Could you check a few things on this model? Use its own coordinates, in mm. A direction names the side the tool comes from. Give positions to 0.01 mm unless a question says otherwise; leave off trailing zeros. Loops run counter-clockwise (first coordinate to the right, second up) from the corner with the lowest first, then second, coordinate; pieces in that order, holes last.
1. For faces 1 (the cylindrical face through (-8.5, 4.2, -13)), 2 (the cylindrical face through (-0.1, 0.5, -11.3)), 3 (the cylindrical face through (-0.111, -0.844, -9.486)), which set-ups out of +Z, -Z, +X, -X, +Y, -Y let a thin tool reach every point of the face, with its end or its side?
2. Thinking about a two-plate mould opening in Y: for faces 4 (the cylindrical face through (-11.51, -3.62, -13.38)), 5 (the flat face through (1, 12, -6.35)), 6 (the conical face through (-0.8, 0.61, -8.11)), which applies, +Y half, -Y half, draft (parallel to the pull), parting line (faces both ways), or undercut?
3. I need wall thicknesses on line 1 along Y through (x, z) = (0, -9.65); line 2 along Y through (x, z) = (0, -13.3) (3 decimals); line 3 along Z through (x, y) = (8.5, -8). Which ranges of each line are inside material? Lowest first, please.
4. Imagine slicing it at A-A (z = -1.25). List the corners of the cut face in (x, y) for me.
5. For P1, Ø3.5, axis at x = -2.5, y = 2.5, coming from the -Z side; P2, Ø5, axis at x = 1.5, z = -15, coming from the -Y side (3 decimals); P3, Ø2, axis at y = 7, z = -15.5, coming from the -X side, each with a flat end and sliding along its axis, tell me the tip position at first contact or that it passes through.
6. Imagine slicing it at B-B (z = -4.25). List the corners of the cut face in (x, y) for me, plus the area to 3 significant figures.
```python
from build123d import *

# Parameters (mm, degrees)
F_6_32_TAPPED_HOLE1_D            = 2.7051
F_6_32_TAPPED_HOLE1_DEPTH        = 9.398
F_6_32_TAPPED_HOLE1_TIP          = 0.81269403
CHAMFER1_SIZE                    = 1.27
CHAMFER1_SIZE2                   = 0.462242198
F_10_32_TAPPED_HOLE2_D           = 4.0386
F_10_32_TAPPED_HOLE2_DEPTH       = 5.9944
F_10_32_TAPPED_HOLE2_CSINK_D     = 5.334
F_10_32_TAPPED_HOLE2_CSINK_ANGLE = 90
F_10_32_TAPPED_HOLE2_TIP         = 1.213317848
FILLET1_R                        = 0.254
CHAMFER2_SIZE                    = 1.27
CHAMFER2_SIZE2                   = 0.340295474


with BuildPart() as part:
    # Sketch1 → Revolve1 (revolve)
    with BuildSketch(Plane(origin=(0, 0, 0), x_dir=(0, 0, -1), z_dir=(1, 0, 0)), mode=Mode.PRIVATE) as revolve1_sk:
        Polygon((0, 0), (0, 13.462), (2.794, 13.462), (2.794, 11.43), (6.35, 11.43), (6.35, 13.462), (10.16, 13.462), (10.16, 12.065), (17.78, 12.065), (17.78, 5.5118), (12.192, 5.5118), (12.192, 0), align=None)
    revolve(revolve1_sk.sketch.rotate(Axis((0, 0, -12.192), (0, 0, 1)), 90), axis=Axis((0, 0, -12.192), (0, 0, 1)))

    # #6-32 Tapped Hole1
    with Locations(Plane(origin=(4.52225484, 6.077033904, -17.78), x_dir=(-1, 0, 0), z_dir=(0, 0, -1))):
        with Locations((-2.626784868, -1.949533904), (4.52225484, -14.332033904), (11.671294548, -1.949533904)):
            Hole(F_6_32_TAPPED_HOLE1_D / 2, depth=F_6_32_TAPPED_HOLE1_DEPTH)
            with Locations((0, 0, -(F_6_32_TAPPED_HOLE1_DEPTH + F_6_32_TAPPED_HOLE1_TIP / 2))):  # 118° drill point
                Cone(0, F_6_32_TAPPED_HOLE1_D / 2, F_6_32_TAPPED_HOLE1_TIP, mode=Mode.SUBTRACT)

    # Chamfer1
    chamfer1_edges = [part.edges().sort_by_distance(p)[0] for p in [
        (5.5118, 0, -17.78),
    ]]
    chamfer1_side = [part.faces().sort_by_distance(p)[0] for p in [
        (5.5118, 0, -14.986),
    ]]
    chamfer(chamfer1_edges, length=CHAMFER1_SIZE, length2=CHAMFER1_SIZE2, reference=chamfer1_side[0])

    # Sketch15 → Church tap on CL (revolve, cut)
    with BuildSketch(Plane(origin=(0, 0, 0), x_dir=(0, 0, -1), z_dir=(1, 0, 0)), mode=Mode.PRIVATE) as church_tap_on_cl_sk:
        Polygon((10.414, 0.508), (17.78, 0.508), (17.78, 0), (0, 0), (0, 2.0193), (6.604, 2.0193), (6.962810512, 1.422139028), (8.532276841, 0.8509), (10.414, 0.8509), align=None)
    revolve(church_tap_on_cl_sk.sketch.rotate(Axis((0, 0, -17.643825074), (0, 0, -1)), 90), axis=Axis((0, 0, -17.643825074), (0, 0, -1)), mode=Mode.SUBTRACT)

    # #10-32 Tapped Hole2
    with Locations(Plane.XY):
        with Locations((0, 0)):
            CounterSinkHole(F_10_32_TAPPED_HOLE2_D / 2, F_10_32_TAPPED_HOLE2_CSINK_D / 2, depth=F_10_32_TAPPED_HOLE2_DEPTH, counter_sink_angle=F_10_32_TAPPED_HOLE2_CSINK_ANGLE)
            with Locations((0, 0, -(F_10_32_TAPPED_HOLE2_DEPTH + F_10_32_TAPPED_HOLE2_TIP / 2))):  # 118° drill point
                Cone(0, F_10_32_TAPPED_HOLE2_D / 2, F_10_32_TAPPED_HOLE2_TIP, mode=Mode.SUBTRACT)

    # Fillet1
    fillet1_edges = [part.edges().sort_by_distance(p)[0] for p in [
        (11.43, 0, -2.794),
        (13.462, 0, -2.794),
        (13.462, 0, -6.35),
        (11.43, 0, -6.35),
    ]]
    fillet(fillet1_edges, radius=FILLET1_R)

    # Chamfer2
    chamfer2_edges = [part.edges().sort_by_distance(p)[0] for p in [
        (12.065, 0, -17.78),
    ]]
    chamfer2_side = [part.faces().sort_by_distance(p)[0] for p in [
        (12.065, 0, -13.97),
    ]]
    chamfer(chamfer2_edges, length=CHAMFER2_SIZE, length2=CHAMFER2_SIZE2, reference=chamfer2_side[0])


solid = part.part
```
Derived:
1. face 1: -Z
1. face 2: +Z, -Z
1. face 3: +Z
2. face 4: parting line
2. face 5: draft
2. face 6: undercut
3. line 1: y = -13.46 to -9.61, -6.9 to -0.85, 0.85 to 13.46
3. line 2: y = -12.065 to -9.608, -6.902 to -5.512, 5.512 to 12.065
3. line 3: z = -17.78 to -6.35, -2.79 to 0
4. outline: circle Ø26.92 at (0, 0); hole circle Ø4.04 at (0, 0)
5. P1: stops at z = -12.19
5. P2: stops at y = -12.065
5. P3: stops at x = -10.47
6. outline: circle Ø22.86 at (0, 0); hole circle Ø4.04 at (0, 0)
6. area: 398 mm2
